Autodesk Inventor part; units mm, degrees
ref_plane "YZ Plane" through (0, 0, 0) normal (1, 0, 0) x (0, 1, 0)
ref_plane "XZ Plane" through (0, 0, 0) normal (0, 1, 0) x (-1, 0, 0)
ref_plane "XY Plane" through (0, 0, 0) normal (0, 0, 1) x (1, 0, 0)
sketch "Sketch1" plane through (0, 0, 0) normal (0, 1, 0) x (-1, 0, 0)
  line L0 (0, 0) -> (-50, 0)
  line L1 (-50, 0) -> (-50, -30)
  line L2 (0, -30) -> (0, 0)
  line L3 (-50, -15) -> (-15, -15) construction
  arc A0 (-11.9, -15) -> (-18.1, -15) centre (-15, -15) ccw
  line L4 (-11.9, -15) -> (-11.9, -30)
  line L5 (-18.1, -15) -> (-18.1, -30)
  line L6 (-50, -30) -> (-18.1, -30)
  line L7 (-11.9, -30) -> (0, -30)
  dimension "d0" = 35
  dimension "d1" = 6.2
  dimension "d2" = 30
  dimension "d3" = 50
extrude "Extrusion1" add sketch "Sketch1" along normal blind 4
sketch "Sketch3" plane through (0, 4, 0) normal (0, 1, 0) x (1, 0, 0)
  line L0 (50, 30) -> (18.1, 30)
  line L1 (30, 30) -> (30, 4)
  line L2 (30, 4) -> (50, 4)
  line L3 (0, 30) -> (0, 0)
  line L4 (26, 30) -> (26, 0)
  line L5 (0, 0) -> (50, 0)
  line L6 (50, 0) -> (50, 30)
  dimension "d12" = 30
  dimension "d13" = 4
  dimension "d14" = 4
extrude "Extrusion3" add sketch "Sketch3" along normal blind 12 contours L1 L2 L6 L5 L4 L0
fillet "Fillet2" radius 2 3 edges at (26, 4, -15) (30, 4, -17) (40, 4, -4)
properties part number "Laptop-ecke-l_3DPrint"
Work out the finished part from the listing and answer in its coordinate system (mm). A direction names the side the tool comes from. Round coordinates to 2 decimals unless told otherwise and drop trailing zeros. Write each loop counter-clockwise with the first axis right and the second up, starting at its lowest first coordinate (ties: lowest second). Pieces come first, ordered by that corner, then holes. Notation, with made-up numbers: M -16,28.5 L 15,28.5 A9 ccw 15,40.5 Z; hole C -17.5,45 d4. An arc over 180 degrees is marked long. Use a Markdown table: item, result.
1) Determine the mould class of faces 1 (the face through (30.57, 4.6, -16.82)), 2 (the face through (18.1, 2, -22)), 3 (the face through (36, 6, 0)) for opening direction X: pulls with the +X half, pulls with the -X half, needs draft (parallel to the pull), parting line crosses it, or undercut.
Taken from the geometry:
| item | result |
|---|---|
| face 1 | pulls with the +X half |
| face 2 | undercut |
| face 3 | needs draft |
2) Consider line 1 (X direction, y = 15, z = -10.75); line 2 (X direction, y = 3.5, z = -18); line 3 (Z direction, x = 33, y = 9.5). Determine where each line is inside the solid, lowest interval first. Write a range as [from, to].
Taken from the geometry:
| item | result |
|---|---|
| line 1 | x = [26, 30] |
| line 2 | x = [0, 11.9], [18.1, 50] |
| line 3 | z = [-4, 0] |
3) Flat-ended cylindrical pins translate along their axes: pin 1 (8 mm diameter, centred on y = 4.5, z = -17.5, fed in from -X); pin 2 (8 mm diameter, centred on y = 10, z = -19, fed in from -X); pin 3 (10 mm diameter, centred on x = 39, z = -17, fed in from +Y); pin 4 (2 mm diameter, centred on y = 8.5, z = -6.5, fed in from +X). Find the tip coordinate at first contact, or state that the pin passes through.
Taken from the geometry:
| item | result |
|---|---|
| pin 1 | stops at x = 0 |
| pin 2 | stops at x = 26 |
| pin 3 | stops at y = 4 |
| pin 4 | stops at x = 30 |
4) The part is cut by section B-B on z = -9.5. Give the vertices of the cut face in (x, y).
Taken from the geometry:
| item | result |
|---|---|
| outline | M 0,0 L 50,0 L 50,4 L 32,4 A2 cw 30,6 L 30,16 L 26,16 L 26,6 A2 cw 24,4 L 0,4 Z |
5) The part is cut by section D-D on y = 9.75. Give the vertices of the cut face in (x, z).
Taken from the geometry:
| item | result |
|---|---|
| outline | M 26,-30 L 30,-30 L 30,-4 L 50,-4 L 50,0 L 26,0 Z |
6) The part is cut by section C-C on x = 34. Give the vertices of the cut face in (y, z).
Taken from the geometry:
| item | result |
|---|---|
| outline | M 0,-30 L 4,-30 L 4,-6 A2 cw 6,-4 L 16,-4 L 16,0 L 0,0 Z |
7) The part is cut by section A-A on z = -18. Give the vertices of the cut face in (x, y).
Taken from the geometry:
| item | result |
|---|---|
| outline | M 0,0 L 11.9,0 L 11.9,4 L 0,4 Z; M 18.1,0 L 50,0 L 50,4 L 32,4 A2 cw 30,6 L 30,16 L 26,16 L 26,6 A2 cw 24,4 L 18.1,4 Z |
8) Which of the six approach directions +Z, -Z, +X, -X, +Y, -Y give full straight-line access (tool end or side, diameter ignored) to faces 4 (the face through (41, 4, -18)), 5 (the face through (0, 2, -15)), 6 (the face through (26, 11, -15)), 7 (the face through (11.9, 2, -22))?
Taken from the geometry:
| item | result |
|---|---|
| face 4 | -Z, +X, +Y |
| face 5 | +Z, -Z, -X, +Y, -Y |
| face 6 | +Z, -Z, -X, +Y |
| face 7 | -Z, +Y, -Y |
